Drawing for the job (mm, zero at the part's lowest x, y, z). Give positions to 0.01 mm unless a question says otherwise; leave off trailing zeros. Order: outer loops, then holes, each group sorted by start corner. A loop starts at its lowest first (then second) coordinate and runs counter-clockwise, first axis right, second up. Notation, with made-up numbers: (31.25, -2.5) - (44.25, -2.5) arc R19 cw to (44.25, 11.5) - close; hole circle Ø4 at (-22.5, 84). An arc over 180 degrees is marked (long way). Use a Markdown table: item, result. Add a question column.
(1) Slice it at B-B (z = 1.15). Write the cut outline in (x, y) (1 decimal), then the cut area to 3 significant figures.
(2) Slice it at D-D (x = 7). Write the cut outline in (y, z).
(3) Wall check: line 1 (Y direction, x = 28, z = 0.45); line 2 (Y direction, x = 29, z = 1) (1 decimal); line 3 (X direction, y = 10.5, z = 0.25) (1 decimal). Give the ranges that are in metal, low to high.
(4) Slice it at A-A (y = 12.7). Write the cut outline in (x, z).
(5) Slice it at C-C (x = 25.5). Write the cut outline in (y, z).
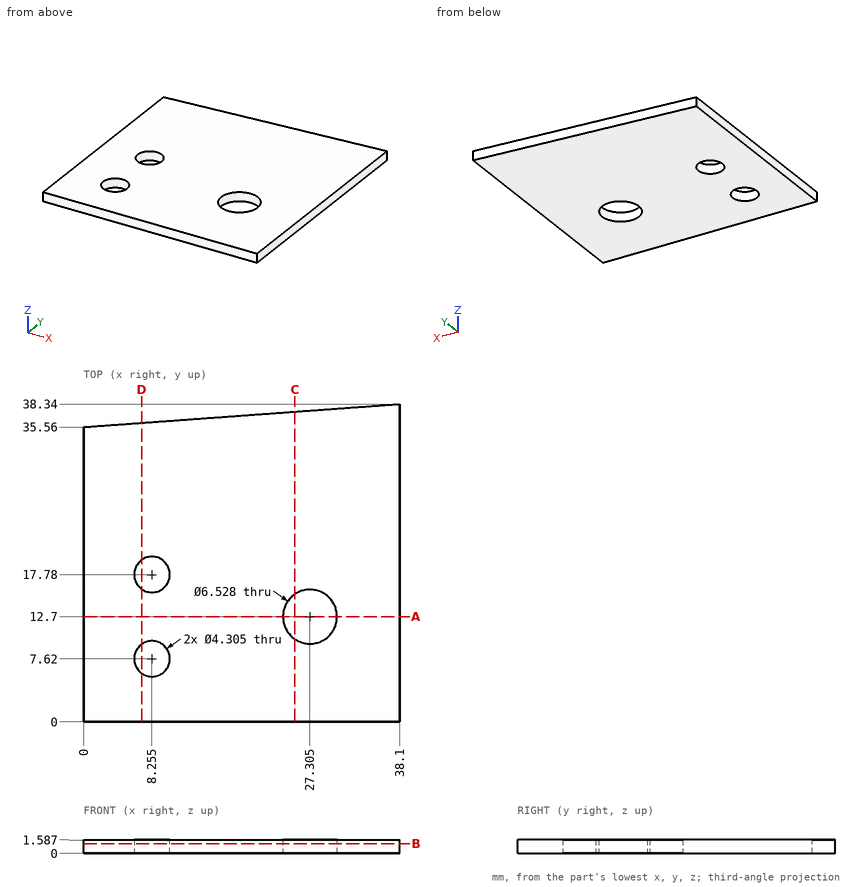
Solution:
| question | item | result |
|---|---|---|
| 1 | outline | (0, 0) - (38.1, 0) - (38.1, 38.3) - (0, 35.6) - close; hole circle Ø4.3 at (8.3, 7.6); hole circle Ø4.3 at (8.3, 17.8); hole circle Ø6.5 at (27.3, 12.7) |
| 1 | area | 1,350 mm2 |
| 2 | outline | (0, 0) - (5.87, 0) - (5.87, 1.59) - (0, 1.59) - close; (9.37, 0) - (16.03, 0) - (16.03, 1.59) - (9.37, 1.59) - close; (19.53, 0) - (36.07, 0) - (36.07, 1.59) - (19.53, 1.59) - close |
| 3 | line 1 | 0 to 9.51, 15.89 to 37.6 |
| 3 | line 2 | 0 to 9.9, 15.5 to 37.7 |
| 3 | line 3 | 0 to 24.9, 29.7 to 38.1 |
| 4 | outline | (0, 0) - (24.04, 0) - (24.04, 1.59) - (0, 1.59) - close; (30.57, 0) - (38.1, 0) - (38.1, 1.59) - (30.57, 1.59) - close |
| 5 | outline | (0, 0) - (9.98, 0) - (9.98, 1.59) - (0, 1.59) - close; (15.42, 0) - (37.42, 0) - (37.42, 1.59) - (15.42, 1.59) - close |
